Autodesk Inventor part; units mm, degrees
ref_plane "YZ Plane" through (0, 0, 0) normal (1, 0, 0) x (0, 1, 0)
ref_plane "XZ Plane" through (0, 0, 0) normal (0, 1, 0) x (-1, 0, 0)
ref_plane "XY Plane" through (0, 0, 0) normal (0, 0, 1) x (1, 0, 0)
sketch "Sketch1" plane through (0, 0, 0) normal (0, 1, 0) x (-1, 0, 0)
  line L0 (0, 0) -> (14, 0)
  line L1 (14, 0) -> (14, -21)
  line L2 (14, -21) -> (0, -21)
  line L3 (0, -21) -> (0, 0)
  circle A0 centre (7, 3) radius 2.65
  circle A1 centre (7, -24) radius 2.65
  circle A2 centre (7, 0) radius 7
  circle A3 centre (7, -21) radius 7
  line L4 (9.65, 1.47) -> (7, -0.06)
  line L5 (7, -0.06) -> (4.35, 1.47)
  line L6 (4.35, 1.47) -> (4.35, 4.53)
  line L7 (4.35, 4.53) -> (7, 6.06)
  line L8 (7, 6.06) -> (9.65, 4.53)
  line L9 (9.65, 4.53) -> (9.65, 1.47)
  line L10 (9.65, -25.53) -> (7, -27.06)
  line L11 (7, -27.06) -> (4.35, -25.53)
  line L12 (4.35, -25.53) -> (4.35, -22.47)
  line L13 (4.35, -22.47) -> (7, -20.94)
  line L14 (7, -20.94) -> (9.65, -22.47)
  line L15 (9.65, -22.47) -> (9.65, -25.53)
  line L16 (14, -10.5) -> (0, -10.5) construction
  circle A4 centre (10.5, -10.5) radius 1.75
  circle A5 centre (3.5, -10.5) radius 1.75
  point P0 (9.65, 3)
  point P1 (9.65, -24)
  dimension "d2" = 5.3
  dimension "d3" = 5.3
  dimension "d0" = 14
  dimension "d1" = 21
  dimension "d4" = 3
  dimension "d5" = 3
  dimension "d6" = 3.5
  dimension "d7" = 3.5
  dimension "d8" = 3.5
  dimension "d9" = 3.5
extrude "Extrusion1" add sketch "Sketch1" along normal blind 3 contours A2 L0 L4 L9 L8 L7 L6 L5 | A2 L1 A3 L3 | L0 L5 L4 A2 | A3 L2 L14 L13 | L2 L13 L12 L11 L10 L15 L14 A3
properties part number "Stationary bracket aligner_3DPrint"
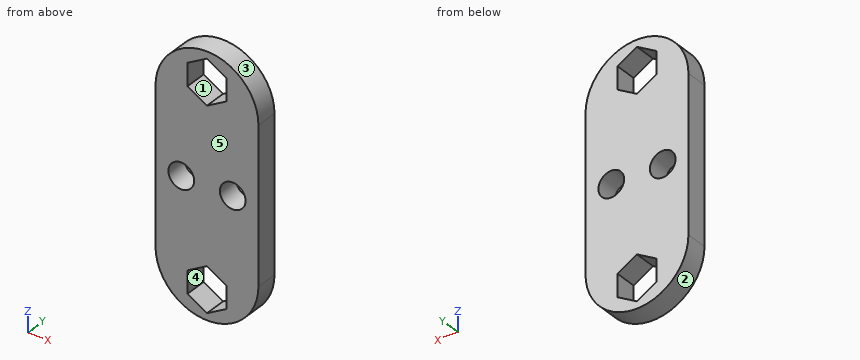
CAD build for the part. Positions are in the model's coordinates, mm. Face numbers are marked on the shaded views. A direction names the side the tool comes from. Coordinates: 2 decimals unless noted, no trailing zeros. Order: outer loops, then holes, each group sorted by start corner. A loop starts at its lowest first (then second) coordinate and runs counter-clockwise, first axis right, second up. Notation, with made-up numbers: (36.5, -18) - (41.5, -18) arc R37 ccw to (41.5, 21) - close; hole circle Ø4 at (-15, 37). An arc over 180 degrees is marked (long way). Answer in a Markdown table with one row per item.
1. 3-axis set-ups, long thin cutter, end or side, ignore diameter. For the marked faces 1 and 2: which of +Z, -Z, +X, -X, +Y, -Y reach the whole face in a straight line?
Answer:
| item | result |
|---|---|
| face 1 | +Y, -Y |
| face 2 | -Z, +Y, -Y |
2. Flat gauge pins, fed straight in: P1, Ø0.9, axis at y = 2, z = 3, coming from the -X side; P2, Ø4, axis at x = -10.5, z = -10.5, coming from the +Y side; P3, Ø1.5, axis at y = 1, z = -23.5, coming from the +X side; P4, Ø3, axis at x = -3.5, z = -10.5, coming from the +Y side. Where does each tip first touch, or does it go through?
Answer:
| item | result |
|---|---|
| P1 | x = -13.52 |
| P2 | y = 3 |
| P3 | x = -0.22 |
| P4 | through |
3. Slice it at B-B, the plane y = 0.9. List the corners of the cut face in (x, z), then the cut area to 3 significant figures.
Answer:
| item | result |
|---|---|
| outline | (-14, -21) arc R7 ccw to (0, -21) - (0, 0) arc R7 ccw to (-14, 0) - close; hole circle Ø3.5 at (-10.5, -10.5); hole (-9.65, -25.53) - (-7, -27.06) - (-4.35, -25.53) - (-4.35, -22.47) - (-7, -20.94) - (-9.65, -22.47) - close; hole (-9.65, 1.47) - (-7, -0.06) - (-4.35, 1.47) - (-4.35, 4.53) - (-7, 6.06) - (-9.65, 4.53) - close; hole circle Ø3.5 at (-3.5, -10.5) |
| area | 380 mm² |
4. Pull direction Z, two halves, no side cores. Call the marked faces 3, 4 and 5: +Z half, -Z half, draft (parallel to the pull), parting line (faces both ways), or undercut.
Answer:
| item | result |
|---|---|
| face 3 | +Z half |
| face 4 | undercut |
| face 5 | draft |
5. Slice it at A-A, the plane z = -10.5. List the corners of the cut face in (x, y), then the cut area to 3 significant figures.
Answer:
| item | result |
|---|---|
| outline | (-14, 0) - (-12.25, 0) - (-12.25, 3) - (-14, 3) - close; (-8.75, 0) - (-5.25, 0) - (-5.25, 3) - (-8.75, 3) - close; (-1.75, 0) - (0, 0) - (0, 3) - (-1.75, 3) - close |
| area | 21.0 mm² |
6. Drill centre lines: L1, parallel to Z at x = -7.75, y = 0.8; L2, parallel to X at y = 1.95, z = -11; L3, parallel to Z at x = -10.5, y = 2. Where is each one in solid material? Low to high. Write a range as from..to.
Answer:
| item | result |
|---|---|
| L1 | -27.96..-26.63, -21.37..0.37, 5.63..6.96 |
| L2 | -14..-12.18, -8.82..-5.18, -1.82..0 |
| L3 | -27.06..-12.25, -8.75..6.06 |
7. Slice it at C-C, the plane z = 5. List the corners of the cut face in (x, y).
Answer:
| item | result |
|---|---|
| outline | (-11.9, 0) - (-8.84, 0) - (-8.84, 3) - (-11.9, 3) - close; (-5.16, 0) - (-2.1, 0) - (-2.1, 3) - (-5.16, 3) - close |
8. Slice it at D-D, the plane x = -6.5. List the corners of the cut face in (y, z).
Answer:
| item | result |
|---|---|
| outline | (0, -27.98) - (3, -27.98) - (3, -26.77) - (0, -26.77) - close; (0, -21.23) - (3, -21.23) - (3, 0.23) - (0, 0.23) - close; (0, 5.77) - (3, 5.77) - (3, 6.98) - (0, 6.98) - close |
